Part model, mm, in its own coordinate system. Face numbers are marked on the shaded views. A direction names the side the tool comes from. Give positions to 0.01 mm unless a question says otherwise; leave off trailing zeros. Write each loop counter-clockwise with the first axis right and the second up, starting at its lowest first coordinate (ties: lowest second). Pieces come first, ordered by that corner, then holes. Notation, with made-up numbers: (26.25, 74) - (85.25, 74) arc R28 cw to (85.25, 112) - close; hole circle Ø7 at (25.5, 75). An arc over 180 degrees is marked (long way). Answer in a Markdown table with one row per item. Add a question column.
1. Which spindle directions (+Z, -Z, +X, -X, +Y, -Y) get a long thin tool onto all of the face, cutting with end or side? Do the marked faces 1, 2 and 3. Say none if no direction does.
2. Pull direction Z, two halves, no side cores. Call the marked faces 4, 5 and 6: released by +Z, released by -Z, zero draft, split by the parting line, or undercut.
3. Band-saw the part on D-D on x = 2.75. Write the cut outline in (y, z), plus the area to 3 significant figures.
4. Band-saw the part on A-A on y = 8. Write the cut outline in (x, z), plus the area to 3 significant figures.
5. Drop flat-ended pins along their axis: pin 1 Ø1 at (y, z) = (24.5, -12) entering from +X; pin 2 Ø1 at (y, z) = (31, -14) entering from +X; pin 3 Ø2.5 at (x, z) = (10, -7.32) entering from +Y; pin 4 Ø3 at (x, y) = (12, 13.5) entering from +Z. Give the stop position or say it passes through.
6. Band-saw the part on C-C on y = 25. Write the cut outline in (x, z), plus the area to 3 significant figures.
7. Probe line 1 along X through (y, z) = (9.5, -7.5); line 2 along X through (y, z) = (7.5, -1.5); line 3 along X through (y, z) = (14, -7.5). List the from-to ranges inside material, lowest first.
8. Band-saw the part on B-B on x = 17.5. Write the cut outline in (y, z), plus the area to 3 significant figures.
```python
from build123d import *

# Parameters (mm, degrees)
EXTRUDE_1_DEPTH        = 40
HOLE_WIZARD_M4_1_D     = 3.3
HOLE_WIZARD_M4_1_DEPTH = 10.1
HOLE_WIZARD_M4_1_TIP   = 0.991420021
HOLE_WIZARD_M4_2_D     = 3.3
HOLE_WIZARD_M4_2_DEPTH = 10.1
HOLE_WIZARD_M4_2_TIP   = 0.991420021
HOLE_WIZARD_M4_3_D     = 3.3
HOLE_WIZARD_M4_3_DEPTH = 10.1
HOLE_WIZARD_M4_3_TIP   = 0.991420021


with BuildPart() as part:
    # 草图1 → 凸台-拉伸1 (new body)
    with BuildSketch(Plane(origin=(0, 0, 0), x_dir=(1, 0, 0), z_dir=(0, 1, 0))):
        Polygon((0, 0), (20, 0), (10, 17.320508076), align=None)
    extrude(amount=EXTRUDE_1_DEPTH)

    # M4 螺纹孔1
    with Locations(Plane(origin=(0, 0, 0), x_dir=(-1, 0, 0), z_dir=(0, -1, 0))):
        with Locations((-10, 7.320508076)):
            Hole(HOLE_WIZARD_M4_1_D / 2, depth=HOLE_WIZARD_M4_1_DEPTH)
            with Locations((0, 0, -(HOLE_WIZARD_M4_1_DEPTH + HOLE_WIZARD_M4_1_TIP / 2))):  # 118° drill point
                Cone(0, HOLE_WIZARD_M4_1_D / 2, HOLE_WIZARD_M4_1_TIP, mode=Mode.SUBTRACT)

    # M4 螺纹孔2
    with Locations(Plane(origin=(0, 40, 0), x_dir=(1, 0, 0), z_dir=(0, 1, 0))):
        with Locations((10, 7.320508076)):
            Hole(HOLE_WIZARD_M4_2_D / 2, depth=HOLE_WIZARD_M4_2_DEPTH)
            with Locations((0, 0, -(HOLE_WIZARD_M4_2_DEPTH + HOLE_WIZARD_M4_2_TIP / 2))):  # 118° drill point
                Cone(0, HOLE_WIZARD_M4_2_D / 2, HOLE_WIZARD_M4_2_TIP, mode=Mode.SUBTRACT)

    # M4 螺纹孔3
    with Locations(Plane(origin=(0, 0, 0), x_dir=(-0.5, 0, 0.866025404), z_dir=(-0.866025404, 0, -0.5))):
        with Locations((-10, 35), (-10, 5)):
            Hole(HOLE_WIZARD_M4_3_D / 2, depth=HOLE_WIZARD_M4_3_DEPTH)
            with Locations((0, 0, -(HOLE_WIZARD_M4_3_DEPTH + HOLE_WIZARD_M4_3_TIP / 2))):  # 118° drill point
                Cone(0, HOLE_WIZARD_M4_3_D / 2, HOLE_WIZARD_M4_3_TIP, mode=Mode.SUBTRACT)


solid = part.part
```
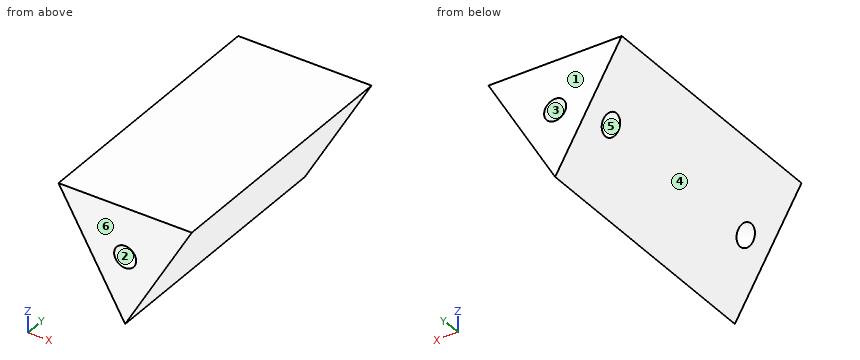
Values:
| question | item | result |
|---|---|---|
| 1 | face 1 | +Z, -Z, +X, -X, +Y |
| 1 | face 2 | -Y |
| 1 | face 3 | +Y |
| 2 | face 4 | released by -Z |
| 2 | face 5 | undercut |
| 2 | face 6 | zero draft |
| 3 | outline | (0, -4.76) - (40, -4.76) - (40, 0) - (0, 0) - close |
| 3 | area | 191 mm² |
| 4 | outline | (0, 0) - (10, -17.32) - (20, 0) - close; hole circle Ø3.3 at (10, -7.32) |
| 4 | area | 165 mm² |
| 5 | pin 1 | stops at x = 13.36 |
| 5 | pin 2 | stops at x = 12.21 |
| 5 | pin 3 | stops at y = 29.66 |
| 5 | pin 4 | stops at z = 0 |
| 6 | outline | (0, 0) - (10, -17.32) - (20, 0) - close |
| 6 | area | 173 mm² |
| 7 | line 1 | x = 4.33 to 8.36, 11.64 to 15.67 |
| 7 | line 2 | x = 0.87 to 19.13 |
| 7 | line 3 | x = 4.33 to 15.67 |
| 8 | outline | (0, -4.33) - (40, -4.33) - (40, 0) - (0, 0) - close |
| 8 | area | 173 mm² |
